Job drawing, mm, ordinate dimensions from the low corner. One solid piece. A direction names the side the tool comes from. Round coordinates to 2 decimals unless told otherwise and drop trailing zeros. Loops run counter-clockwise (first coordinate to the right, second up) from the corner with the lowest first, then second, coordinate; pieces in that order, holes last. Notation, with made-up numbers: M 68,86.25 L 120,86.25 A20 cw 120,119.25 Z; hole C -31,66.5 d9. An arc over 180 degrees is marked long. Write each question's results on one line, items separated by ' | '. Start each with the question number.
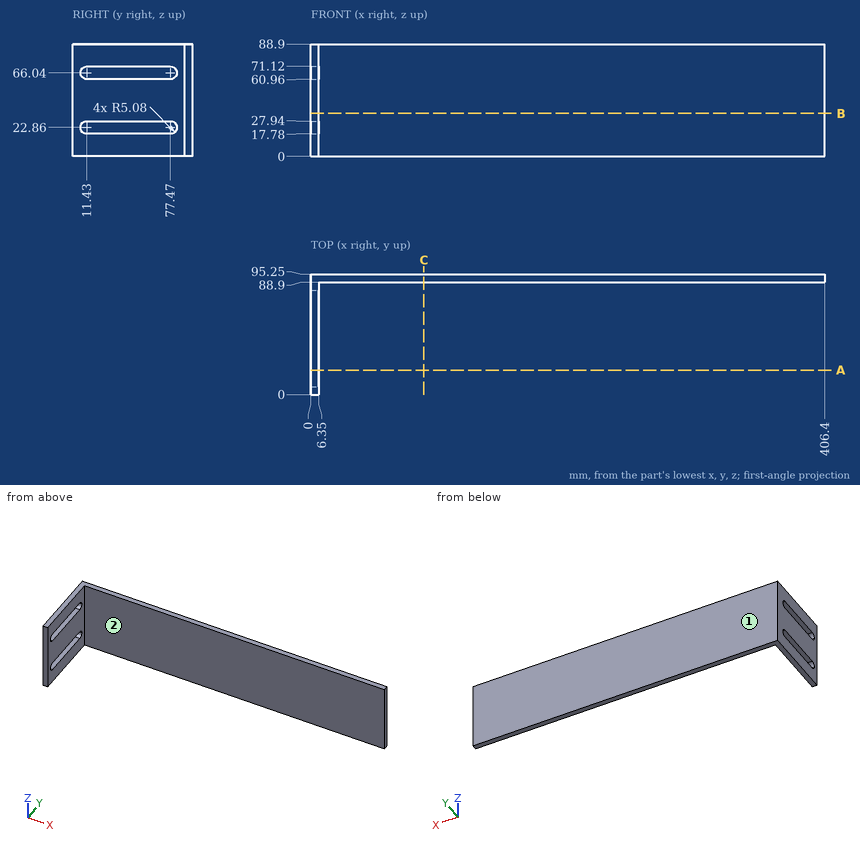
Item 1: Saw through at B-B, the plane z = 34. Give the cut face in (x, y), then the cut area to 3 significant figures.
Item 2: Tool access for the marked faces 1 and 2: list every direction of +Z, -Z, +X, -X, +Y, -Y with a clear straight run to the whole face (end or side of a thin tool).
Item 3: Saw through at A-A, the plane y = 19.5. Give the cut face in (x, z), then the cut area to 3 significant figures.
Item 4: Drop flat-ended pins along their axis: pin 1 (4 mm diameter, centred on x = 335, z = 36, fed in from -Y); pin 2 (10 mm diameter, centred on y = 23, z = 48.5, fed in from +X). Give the stop position or say it passes through.
Item 5: Drill centre lines: line 1 along Y through (x, z) = (168.5, 77.5); line 2 along X through (y, z) = (29, 83). Where is each one in solid material? Low to high. Write a range as [from, to].
Item 6: Saw through at C-C, the plane x = 89.5. Give the cut face in (y, z).
Working result:
1) outline: M 0,0 L 6.35,0 L 6.35,88.9 L 406.4,88.9 L 406.4,95.25 L 0,95.25 Z | area: 3,150 mm²
2) face 1: +Z, -Z, +X, -X, +Y | face 2: +Z, -Z, +X, -Y
3) outline: M 0,0 L 6.35,0 L 6.35,17.78 L 0,17.78 Z; M 0,27.94 L 6.35,27.94 L 6.35,60.96 L 0,60.96 Z; M 0,71.12 L 6.35,71.12 L 6.35,88.9 L 0,88.9 Z | area: 435 mm²
4) pin 1: stops at y = 88.9 | pin 2: stops at x = 6.35
5) line 1: y = [88.9, 95.25] | line 2: x = [0, 6.35]
6) outline: M 88.9,0 L 95.25,0 L 95.25,88.9 L 88.9,88.9 Z
